For this review, take the finished solid that the model builds, in its own axes (mm). Face numbers are marked on the shaded views. A direction names the side the tool comes from. Coordinates: 2 decimals unless noted, no trailing zeros. Loops run counter-clockwise (first coordinate to the right, second up) from the corner with the lowest first, then second, coordinate; pieces in that order, holes last. Notation, with made-up numbers: (68, 84.25) -> (73, 84.25) arc R12 cw to (73, 105.25) -> close; hole circle Ø6 at (38.5, 2). An arc over 180 degrees is marked (long way). Use a Markdown table: item, result.
from build123d import *

# Parameters (mm, degrees)
SKETCH1_W           = 20
SKETCH1_H           = 20
EXTRUDE1_DEPTH      = 1
SKETCH2_W           = 20
SKETCH2_H           = 20
EXTRUDE2_DEPTH      = 1.5
EXTRUDE2_TAPER      = 75
SKETCH3_W           = 3
SKETCH3_H           = 4
EXTRUDE3_DEPTH      = 2
EXTRUDE_THIN1_DEPTH = 1.5
MOVE_FACE1_BY       = 1
MOVE_FACE1_2_BY     = 1
MOVE_FACE1_3_BY     = 1
SKETCH5_W           = 26.322025843
SKETCH5_H           = 24.141830142
CUT_EXTRUDE1_DEPTH  = 10


with BuildPart() as part:
    # Sketch1 → Extrude1 (new body)
    with BuildSketch(Plane(origin=(0, 0, 0), x_dir=(1, 0, 0), z_dir=(0, 1, 0))):
        Rectangle(SKETCH1_W, SKETCH1_H)
    extrude(amount=EXTRUDE1_DEPTH)

    # Sketch2 → Extrude2 (add)
    with BuildSketch(Plane(origin=(0, 1, 0), x_dir=(-1, 0, 0), z_dir=(0, 1, 0))):
        Rectangle(SKETCH2_W, SKETCH2_H)
    extrude(amount=EXTRUDE2_DEPTH, taper=EXTRUDE2_TAPER)

    # Sketch3 → Extrude3 (add, symmetric)
    with BuildSketch(Plane.XY):
        with Locations((-2.901923789, 4.5)):
            Rectangle(SKETCH3_W, SKETCH3_H)
    extrude(amount=EXTRUDE3_DEPTH, both=True)

    # Sketch4 → Extrude-Thin1 (add, symmetric)
    with BuildSketch(Plane.XY):
        with BuildLine():
            Line((-1.401923789, 6.5), (-1.401923789, 6.7))
            ThreePointArc((-1.401923789, 6.7), (3.719396555, 8.821320344), (1.598076211, 3.7))
            Line((1.598076211, 3.7), (-6.87859684, 3.7))
            Line((-6.87859684, 3.7), (-6.87859684, 2.7))
            Line((-6.87859684, 2.7), (1.598076211, 2.7))
            ThreePointArc((1.598076211, 2.7), (4.426503336, 9.528427125), (-2.401923789, 6.7))
            Line((-2.401923789, 6.7), (-2.401923789, 6.5))
            Line((-2.401923789, 6.5), (-1.401923789, 6.5))
        make_face()
    extrude(amount=EXTRUDE_THIN1_DEPTH, both=True)

    # Move Face1: a face moved inward by 1.0
    extrude(part.faces().sort_by_distance((-2.901923789, 4.5, 2))[0], amount=MOVE_FACE1_BY, dir=(0, 0, -1), mode=Mode.SUBTRACT)

    # Move Face1 2: a face moved inward by 1.0
    extrude(part.faces().sort_by_distance((1.598076211, 3.5, 1.5))[0], amount=MOVE_FACE1_2_BY, dir=(0, 0, -1), mode=Mode.SUBTRACT)

    # Move Face1 3: a face moved inward by 1.0
    extrude(part.faces().sort_by_distance((-5.640260314, 3.2, 1.5))[0], amount=MOVE_FACE1_3_BY, dir=(0, 0, -1), mode=Mode.SUBTRACT)

    # Sketch5 → Cut-Extrude1 (cut)
    with BuildSketch(Plane(origin=(0, 2.5, 0), x_dir=(1, 0, 0), z_dir=(0, 1, 0))):
        with Locations((0.290185678, -1.072850133)):
            Rectangle(SKETCH5_W, SKETCH5_H)
    extrude(amount=-CUT_EXTRUDE1_DEPTH, mode=Mode.SUBTRACT)


solid = part.part
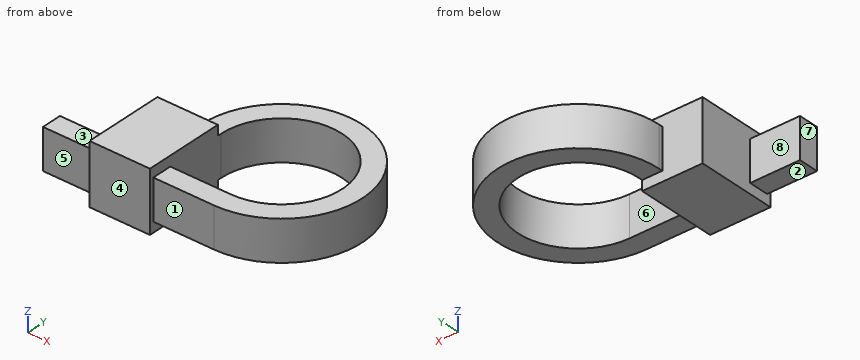
(1) For pin 1 Ø1 at (x, z) = (-6, -0.5) entering from +Y; pin 2 Ø1.6 at (x, z) = (0, -0.5) entering from -Y; pin 3 Ø1.6 at (x, z) = (0, -1) entering from +Y; pin 4 Ø1.6 at (x, z) = (-5, -0.5) entering from -Y, all flat-tipped, find the tip position at first contact; note any pin that passes through.
Found:
| item | result |
|---|---|
| pin 1 | stops at y = 3.7 |
| pin 2 | stops at y = 2.7 |
| pin 3 | stops at y = 10.62 |
| pin 4 | stops at y = 2.5 |
(2) For line 1 along Y through (x, z) = (-2.75, 0.4); line 2 along Z through (x, y) = (-1.75, 7.75); line 3 along Y through (x, z) = (-0.25, -0.7), list the stretches that pass through material, from the lowest coordinate up.
Found:
| item | result |
|---|---|
| line 1 | y = 2.5 to 6.5 |
| line 2 | z = -1.5 to 0.5 |
| line 3 | y = 2.7 to 3.7, 9.06 to 10.25 |
(3) Mouldability with a two-part tool opening along X and no side actions: class the marked faces 6, 7 and 8 as pulls with the +X half, pulls with the -X half, needs draft (parallel to the pull), parting line crosses it, or undercut.
Found:
| item | result |
|---|---|
| face 6 | undercut |
| face 7 | pulls with the -X half |
| face 8 | needs draft |
(4) Take a section at D-D on x = -4. Write out the cut boundary in (y, z), plus the area to 3 significant figures.
Found:
| item | result |
|---|---|
| outline | (2.5, -2) -> (6.5, -2) -> (6.5, 1) -> (2.5, 1) -> close |
| area | 12.0 mm^2 |
(5) Take a section at C-C on x = -0.25. Write out the cut boundary in (y, z).
Found:
| item | result |
|---|---|
| outline | (2.7, -1.5) -> (3.7, -1.5) -> (3.7, 0.5) -> (2.7, 0.5) -> close; (9.06, -1.5) -> (10.25, -1.5) -> (10.25, 0.5) -> (9.06, 0.5) -> close |
(6) Take a section at B-B on y = 7.25. Write out the cut boundary in (x, z), plus the area to 3 significant figures.
Found:
| item | result |
|---|---|
| outline | (-2.36, -1.5) -> (-1.35, -1.5) -> (-1.35, 0.5) -> (-2.36, 0.5) -> close; (4.55, -1.5) -> (5.56, -1.5) -> (5.56, 0.5) -> (4.55, 0.5) -> close |
| area | 4.05 mm^2 |
(7) For the marked faces 1, 2, 3, 4 and 5, list the 3-axis set-ups (+Z, -Z, +X, -X, +Y, -Y) from which the entire face can be reached by the end or side of a thin tool; tool diameter is ignored.
Found:
| item | result |
|---|---|
| face 1 | +Z, -Z, +X, -Y |
| face 2 | -Z, -X, +Y, -Y |
| face 3 | +Z, -X, +Y, -Y |
| face 4 | +Z, -Z, +X, -X, -Y |
| face 5 | +Z, -Z, -X, -Y |
(8) Take a section at A-A on z = -0.05. Write out the cut boundary in (x, y).
Found:
| item | result |
|---|---|
| outline | (-6.88, 2.7) -> (-4.4, 2.7) -> (-4.4, 2.5) -> (-1.4, 2.5) -> (-1.4, 2.7) -> (1.6, 2.7) arc R4 ccw (long way) to (-2.4, 6.7) -> (-2.4, 6.5) -> (-4.4, 6.5) -> (-4.4, 3.7) -> (-6.88, 3.7) -> close; hole (-1.4, 3.7) -> (1.6, 3.7) arc R3 ccw (long way) to (-1.4, 6.7) -> close |
